from build123d import *

# Parameters (mm, degrees)
SZKIC1_W                    = 45
SZKIC1_H                    = 21
SZKIC1_W_2                  = 41
SZKIC1_H_2                  = 17
DODANIE_WYCI_GNI_CIE1_DEPTH = 10
SZKIC2_W                    = 14.5
SZKIC2_H                    = 27.2
SZKIC2_W_2                  = 10.5
SZKIC2_H_2                  = 23.2
DODANIE_WYCI_GNI_CIE2_DEPTH = 3
DODANIE_WYCI_GNI_CIE3_START = -14.5
DODANIE_WYCI_GNI_CIE3_DEPTH = 14.5


with BuildPart() as part:
    # Szkic1 → Dodanie-wyciągnięcie1 (new body)
    with BuildSketch(Plane.XY):
        with Locations((18.754452903, 41.181022194)):
            Rectangle(SZKIC1_W, SZKIC1_H)
        with Locations((18.754452903, 41.181022194)):
            Rectangle(SZKIC1_W_2, SZKIC1_H_2, mode=Mode.SUBTRACT)
    extrude(amount=DODANIE_WYCI_GNI_CIE1_DEPTH)

    # Szkic2 → Dodanie-wyciągnięcie2 (add)
    with BuildSketch(Plane.XY.offset(10)):
        with Locations((18.754452903, 41.181022194)):
            Rectangle(SZKIC2_W, SZKIC2_H)
        with Locations((18.754452903, 41.181022194)):
            Rectangle(SZKIC2_W_2, SZKIC2_H_2, mode=Mode.SUBTRACT)
    extrude(amount=DODANIE_WYCI_GNI_CIE2_DEPTH)

    # Szkic3 → Dodanie-wyciągnięcie3 (add)
    with BuildSketch(Plane(origin=(26.004452903, 0, 0), x_dir=(0, 0, -1), z_dir=(1, 0, 0)).offset(DODANIE_WYCI_GNI_CIE3_START)):
        with BuildLine():
            Line((-10, 54.781022194), (-10, 51.681022194))
            Line((-10, 51.681022194), (-6.9, 51.681022194))
            add(Edge.make_bspline(
                [(-6.9, 51.681022194), (-10, 51.681022194), (-10, 54.781022194)],
                knots=[0, 0, 0, 1, 1, 1], degree=2))
        make_face()
        with BuildLine():
            Line((-10, 27.581022194), (-10, 30.681022194))
            Line((-10, 30.681022194), (-6.9, 30.681022194))
            add(Edge.make_bspline(
                [(-10, 27.581022194), (-10, 30.681022194), (-6.9, 30.681022194)],
                knots=[0, 0, 0, 1, 1, 1], degree=2))
        make_face()
    extrude(amount=DODANIE_WYCI_GNI_CIE3_DEPTH)


solid = part.part
CAD build for the part. Positions are in the model's coordinates, mm. A direction names the side the tool comes from. Give positions to 0.01 mm unless a question says otherwise; leave off trailing zeros. Write each loop counter-clockwise with the first axis right and the second up, starting at its lowest first coordinate (ties: lowest second). Pieces come first, ordered by that corner, then holes. Notation, with made-up numbers: (59.5, 26) -> (93.5, 26) arc R7 ccw to (93.5, 32) -> close; hole circle Ø1 at (-13.5, 37). An arc over 180 degrees is marked (long way). Return JSON: item names as keys, results as strings.
Item 1: Band-saw the part on D-D (y = 51). List the corners of the cut face in (x, z).
Answer below:
{"outline": "(-3.75, 0) -> (41.25, 0) -> (41.25, 10) -> (26, 10) -> (26, 13) -> (24, 13) -> (24, 10) -> (13.5, 10) -> (13.5, 13) -> (11.5, 13) -> (11.5, 10) -> (-3.75, 10) -> close"}
Item 2: Band-saw the part on B-B (x = 1.5). List the corners of the cut face in (y, z), then the cut area to 3 significant figures.
Answer below:
{"outline": "(30.68, 0) -> (32.68, 0) -> (32.68, 10) -> (30.68, 10) -> close; (49.68, 0) -> (51.68, 0) -> (51.68, 10) -> (49.68, 10) -> close", "area": "40.0 mm2"}
Item 3: Drop flat-ended pins along their axis: pin 1 (1.6 mm diameter, centred on x = 20.5, y = 51.5, fed in from +Z); pin 2 (1.6 mm diameter, centred on x = 12.5, y = 39.5, fed in from -Z); pin 3 (0.9 mm diameter, centred on y = 40, z = 12, fed in from -X). Give the stop position or say it passes through.
Answer below:
{"pin 1": "stops at z = 10", "pin 2": "stops at z = 10", "pin 3": "stops at x = 11.5"}
Item 4: Two-plate mould, pull along X, no slides. Class faces 4 (the flat face through (19, 50, 0)), 5 (the flat face through (24.004, 41, 11)), 6 (the flat face through (18, 49.681, 5)), 7 (the flat face through (41.254, 41, 5)): +X half, -X half, draft (parallel to the pull), parting line (faces both ways), or undercut.
Answer below:
{"face 4": "draft", "face 5": "undercut", "face 6": "undercut", "face 7": "+X half"}
Item 5: Band-saw the part on A-A (y = 39.5). List the corners of the cut face in (x, z), then the cut area to 3 significant figures.
Answer below:
{"outline": "(-3.75, 0) -> (-1.75, 0) -> (-1.75, 10) -> (-3.75, 10) -> close; (11.5, 10) -> (13.5, 10) -> (13.5, 13) -> (11.5, 13) -> close; (24, 10) -> (26, 10) -> (26, 13) -> (24, 13) -> close; (39.25, 0) -> (41.25, 0) -> (41.25, 10) -> (39.25, 10) -> close", "area": "52.0 mm2"}
Item 6: Band-saw the part on C-C (z = 5). List the corners of the cut face in (x, y), then the cut area to 3 significant figures.
Answer below:
{"outline": "(-3.75, 30.68) -> (41.25, 30.68) -> (41.25, 51.68) -> (-3.75, 51.68) -> close; hole (-1.75, 32.68) -> (39.25, 32.68) -> (39.25, 49.68) -> (-1.75, 49.68) -> close", "area": "248 mm2"}
Item 7: Tool access for faces 1 (the flat face through (-2, 40, 10)), 2 (the flat face through (19, 31, 10)), 3 (the flat face through (-1.746, 41, 5)): list every direction of +Z, -Z, +X, -X, +Y, -Y with a clear straight run to the whole face (end or side of a thin tool).
Answer below:
{"face 1": "+Z, -X, +Y, -Y", "face 2": "+Z", "face 3": "+Z, -Z"}
Item 8: Drill centre lines: probe 1 along X at (y, z) = (30.5, 11); probe 2 along Y at (x, z) = (0, 3.5); probe 3 along X at (y, z) = (36.5, 3.25). Where is each one in solid material? Low to high.
Answer below:
{"probe 1": "x = 11.5 to 13.5, 24 to 26", "probe 2": "y = 30.68 to 32.68, 49.68 to 51.68", "probe 3": "x = -3.75 to -1.75, 39.25 to 41.25"}
